from build123d import *

# Parameters (mm, degrees)
BOX001_W     = 18.46
BOX001_H     = 14.26
BOX001_DEPTH = 1
BOX_W        = 13.42
BOX_H        = 10.02
BOX_DEPTH    = 0.1


with BuildPart() as obj1:
    # Box001 → Box001 (new body)
    with BuildSketch(Plane.XY):
        with Locations((9.23, 7.13)):
            Rectangle(BOX001_W, BOX001_H)
    extrude(amount=BOX001_DEPTH)


with BuildPart() as display:
    # Box → Box (new body)
    with BuildSketch(Plane(origin=(2.52, 2.6, 1), x_dir=(1, 0, 0), z_dir=(0, 0, 1))):
        with Locations((6.71, 5.01)):
            Rectangle(BOX_W, BOX_H)
    extrude(amount=BOX_DEPTH)

    # Fusion: union obj1
    add(obj1.part)


solid = display.part
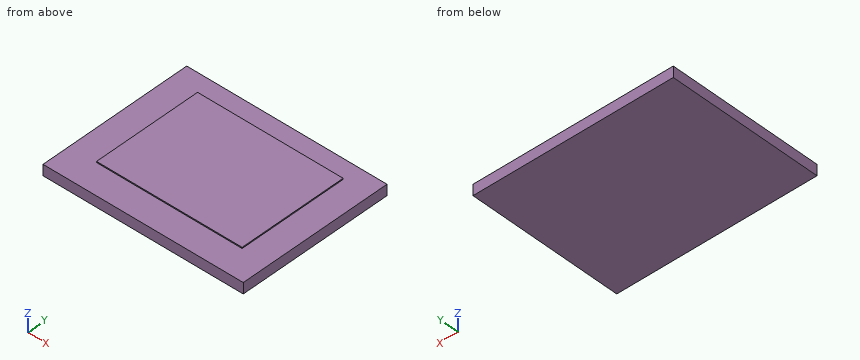
Here's how the part is built. I have some questions about the finished solid (model axes, mm). Round coordinates to 2 decimals unless told otherwise and drop trailing zeros. Loops run counter-clockwise (first coordinate to the right, second up) from the corner with the lowest first, then second, coordinate; pieces in that order, holes last.
1. If we section it at A-A on x = 3.75: Write out the boundary of the cut face in (y, z).
Answer list:
outline: (0, 0) - (14.26, 0) - (14.26, 1) - (12.62, 1) - (12.62, 1.1) - (2.6, 1.1) - (2.6, 1) - (0, 1) - close
2. If I drill on line 1 along Z through (x, y) = (15.25, 2.5), over which ranges is the centre line in solid material (lowest first)?
Answer list:
line 1: z = 0 to 1
3. If we section it at C-C on x = 17.25: Write out the boundary of the cut face in (y, z), plus the area to 3 significant figures.
Answer list:
outline: (0, 0) - (14.26, 0) - (14.26, 1) - (0, 1) - close
area: 14.3 mm2
4. If we section it at B-B on y = 8.25: Write out the boundary of the cut face in (x, z).
Answer list:
outline: (0, 0) - (18.46, 0) - (18.46, 1) - (15.94, 1) - (15.94, 1.1) - (2.52, 1.1) - (2.52, 1) - (0, 1) - close
